Source: CAD feature listing. Evaluate the final solid. Frame: model axes, mm. A direction names the side the tool comes from. Give positions to 0.01 mm unless a question says otherwise; leave off trailing zeros. Loops run counter-clockwise (first coordinate to the right, second up) from the corner with the lowest first, then second, coordinate; pieces in that order, holes last. Notation, with made-up numbers: (33.5, 35) - (74.5, 35) arc R22 cw to (74.5, 63) - close; hole circle Ø3 at (72, 8.25). An arc over 180 degrees is marked (long way). Write each question's results on one line, items separated by ' | '. Start each with the question number.
(1) Reachability of faces 4 (the cylindrical face through (27.614, -11.205, 221.613)), 5 (the cylindrical face through (-49.45, 23.86, -48.18)), 6 (the flat face through (-39, -49.763, 127)) from +Z, -Z, +X, -X, +Y, -Y: full face, straight path, thin tool, end or side. Return the list, or none.
(2) Cut plane B-B on x = 10.5. Give the number of separate pieces and of enclosed holes in the cut face, then the cut area to 3 significant figures.
(3) Contact query for flat-ended pins moving along their axis: pin 1 (10 mm diameter, centred on x = 24, z = 237.5, fed in from +Y); pin 2 (5 mm diameter, centred on y = -4, z = 168, fed in from +X); pin 3 (1 mm diameter, centred on x = 53.5, y = -15, fed in from +Z). Output: stop coordinate, or through.
(4) Material intervals for line 1 along X through (y, z) = (20, 156.5); line 2 along Z through (x, y) = (-36, -55); line 3 along X through (y, z) = (12, 121.5), sorted ascending. Write a range as [from, to].
(5) Pull-direction query (Y, two-part tool) for faces 1 (the flat face through (31.978, -11, 124)), 2 (the cylindrical face through (52.096, -13.097, -48.175)), 3 (the flat face through (-62.829, -68.294, -35.434)); classes: pulls with the +Y half, pulls with the -Y half, needs draft (parallel to the pull), parting line crosses it, or undercut.
(6) Cut plane A-A on z = 124.5. Return the cut outline in (x, y).
(7) Cut plane C-C on y = -2.5. Return the cut outline in (x, z), then the cut area to 3 significant figures.
from build123d import *

# Parameters (mm, degrees)
RESSALTO_EXTRUS_O1_DEPTH             = 250
ESCALA1_SCALE                        = 1.5
AL_VIOS_SUPERIOR_INFERIOR_DEPTH      = 0.1
AL_VIOS_SUPERIOR_INFERIOR_DEPTH_BACK = 265
AL_VIOS_SUPERIOR_INFERIOR_START      = -55
AL_VIO_CENTRAL_DEPTH                 = 342.991467302
ESBO_O7_R                            = 40
REBAIXO_ROLAMENTO_PAI_DEPTH          = 46
ESBO_O7_3_R                          = 25
REBAIXO_ROLAMENTO_FILHO_DEPTH        = 395.297005295
FURO_START                           = -329
FURO_EIXO_ARMA_FILHO_DEPTH           = 46
FUROS_POLIA_PAI_D                    = 8.5
FUROS_POLIA_PAI_DEPTH                = 27.5
FUROS_POLIA_PAI_CSINK_D              = 10.05
FUROS_POLIA_PAI_CSINK_ANGLE          = 90
FUROS_POLIA_PAI_TIP                  = 2.553657631
FUROS_POLIA_FILHO_D                  = 8.5
FUROS_POLIA_FILHO_DEPTH              = 27.5
FUROS_POLIA_FILHO_CSINK_D            = 10.05
FUROS_POLIA_FILHO_CSINK_ANGLE        = 90
FUROS_POLIA_FILHO_TIP                = 2.553657631


with BuildPart() as part:
    # Esboço1 → Ressalto-extrusão1 (new body)
    with BuildSketch(Plane.XY):
        with BuildLine():
            Line((64.316370752, 0), (63.337395385, -14))
            Line((63.337395385, -14), (54.810070893, -37.42863149))
            Line((54.810070893, -37.42863149), (-37.189929107, -52))
            Line((-37.189929107, -52), (-49.547157766, -47.50233659))
            Line((-49.547157766, -47.50233659), (-58, -37.42863149))
            Line((-58, -37.42863149), (-58, 9.144452309))
            Line((-58, 9.144452309), (-49.934391816, 20.66333456))
            Line((-49.934391816, 20.66333456), (-37.189929107, 26.60617512))
            Line((-37.189929107, 26.60617512), (29.770815295, 20.747869084))
            Line((29.770815295, 20.747869084), (35.181577398, 9.144452309))
            ThreePointArc((35.181577398, 9.144452309), (42.631493482, 1.085178494), (53.376629903, -1.149813096))
            Line((53.376629903, -1.149813096), (64.316370752, 0))
        make_face()
    extrude(amount=RESSALTO_EXTRUS_O1_DEPTH)


with BuildPart() as part_1:
    # Escala1: scaled about (-4.187287107, -12.759804583, 125)
    add(part.part.scale(ESCALA1_SCALE).moved(Location((2.093643554, 6.379902291, -62.5))))

    # Esboço4 → Alívios superior / inferior (cut, two sides: drawn at the far end of the back side and taken through both)
    with BuildSketch(Plane(origin=(0, 0, -62.5), x_dir=(-1, 0, 0), z_dir=(0, 0, -1)).offset(AL_VIOS_SUPERIOR_INFERIOR_START - AL_VIOS_SUPERIOR_INFERIOR_DEPTH_BACK)):
        Polygon((-46.749866496, 37.501705917), (-51.978360206, 26.289164972), (80.570262297, 26.289164972), (72.807944171, 37.374904131), (53.691250107, 46.289164972), align=None)
        Polygon((72.227093095, -64.873602594), (84.906356446, -49.763044944), (-84.308749893, -49.763044944), (53.691250107, -71.620097709), align=None)
    extrude(amount=AL_VIOS_SUPERIOR_INFERIOR_DEPTH + AL_VIOS_SUPERIOR_INFERIOR_DEPTH_BACK, mode=Mode.SUBTRACT)

    # Esboço15 → Alívio Central (cut, through all)
    with BuildSketch(Plane(origin=(0, 26.289164972, 0), x_dir=(1, 0, 0), z_dir=(0, 1, 0))):
        with BuildLine():
            Line((-10.570262297, -17.4), (6.978360206, -17.4))
            ThreePointArc((6.978360206, -17.4), (24.656029736, -24.72233047), (31.978360206, -42.4))
            Line((31.978360206, -42.4), (31.978360206, -207.5))
            ThreePointArc((31.978360206, -207.5), (24.656029736, -225.17766953), (6.978360206, -232.5))
            Line((6.978360206, -232.5), (-10.570262297, -232.5))
            ThreePointArc((-10.570262297, -232.5), (-28.247931827, -225.17766953), (-35.570262297, -207.5))
            Line((-35.570262297, -207.5), (-35.570262297, -42.4))
            ThreePointArc((-35.570262297, -42.4), (-28.247931827, -24.72233047), (-10.570262297, -17.4))
        make_face()
    extrude(amount=-AL_VIO_CENTRAL_DEPTH, mode=Mode.SUBTRACT)

    # Esboço7 → Rebaixo rolamento (Pai) (cut)
    with BuildSketch(Plane.XY.offset(312.5)):
        with Locations((-1.158298377, -13.283920248)):
            Circle(ESBO_O7_R)
    extrude(amount=-REBAIXO_ROLAMENTO_PAI_DEPTH, mode=Mode.SUBTRACT)

    # Esboço7<3> → Rebaixo rolamento (Filho) (cut, through all)
    with BuildSketch(Plane.XY.offset(312.5)):
        with Locations((-1.158298377, -13.283920248)):
            Circle(ESBO_O7_3_R)
    extrude(amount=-REBAIXO_ROLAMENTO_FILHO_DEPTH, mode=Mode.SUBTRACT)

    # Esboço7 → Furo eixo arma (Filho) (cut)
    with BuildSketch(Plane.XY.offset(312.5).offset(FURO_START)):
        with Locations((-1.158298377, -13.283920248)):
            Circle(ESBO_O7_R)
    extrude(amount=-FURO_EIXO_ARMA_FILHO_DEPTH, mode=Mode.SUBTRACT)

    # Furos Polia (Pai)
    with Locations(Plane.XY.offset(312.5)):
        with Locations((56.341701623, -13.283920248), (-45.205853857, 23.676367309), (-58.623505242, -11.283920248), (-48.259540924, -46.264565338), (51.370565437, -36.671277225)):
            CounterSinkHole(FUROS_POLIA_PAI_D / 2, FUROS_POLIA_PAI_CSINK_D / 2, depth=FUROS_POLIA_PAI_DEPTH, counter_sink_angle=FUROS_POLIA_PAI_CSINK_ANGLE)
            with Locations((0, 0, -(FUROS_POLIA_PAI_DEPTH + FUROS_POLIA_PAI_TIP / 2))):  # 118° drill point
                Cone(0, FUROS_POLIA_PAI_D / 2, FUROS_POLIA_PAI_TIP, mode=Mode.SUBTRACT)

    # Furos Polia (Filho)
    with Locations(Plane(origin=(0, 0, -62.5), x_dir=(-1, 0, 0), z_dir=(0, 0, -1))):
        with Locations((45.205853857, 23.676367309), (58.623505242, -11.283920248), (48.259540924, -46.264565338), (-51.370565437, -36.671277225), (-56.341701623, -13.283920248)):
            CounterSinkHole(FUROS_POLIA_FILHO_D / 2, FUROS_POLIA_FILHO_CSINK_D / 2, depth=FUROS_POLIA_FILHO_DEPTH, counter_sink_angle=FUROS_POLIA_FILHO_CSINK_ANGLE)
            with Locations((0, 0, -(FUROS_POLIA_FILHO_DEPTH + FUROS_POLIA_FILHO_TIP / 2))):  # 118° drill point
                Cone(0, FUROS_POLIA_FILHO_D / 2, FUROS_POLIA_FILHO_TIP, mode=Mode.SUBTRACT)


solid = part_1.part
Ans:
1) face 4: +Y, -Y | face 5: -Z | face 6: +X, -X, -Y
2) separate pieces: 4 | enclosed holes: 0 | area: 5,000 mm^2
3) pin 1: y = 26.29 | pin 2: x = 98.02 | pin 3: z = 284.74
4) line 1: [-84.91, -35.57], [31.98, 54.91] | line 2: [-62.5, -7.6], [257.5, 312.5] | line 3: [-84.91, -35.57], [31.98, 60.67]
5) face 1: needs draft | face 2: undercut | face 3: pulls with the -Y half
6) outline: (-84.91, -49.76) - (-35.57, -49.76) - (-35.57, 26.29) - (-80.57, 26.29) - (-84.91, 20.1) - close; (31.98, -49.76) - (84.31, -49.76) - (97.1, -14.62) - (98.57, 6.38) - (82.16, 4.66) arc R27 cw to (54.87, 20.1) - (51.98, 26.29) - (31.98, 26.29) - close
7) outline: (-84.91, -62.5) - (-39.68, -62.5) - (-39.68, -16.5) - (-23.71, -16.5) - (-23.71, 21.13) arc R25 cw to (-35.57, 42.4) - (-35.57, 207.5) arc R25 cw to (-23.71, 228.77) - (-23.71, 266.5) - (-39.68, 266.5) - (-39.68, 312.5) - (-84.91, 312.5) - close; (21.4, -16.5) - (37.36, -16.5) - (37.36, -62.5) - (97.95, -62.5) - (97.95, 312.5) - (37.36, 312.5) - (37.36, 266.5) - (21.4, 266.5) - (21.4, 227.92) arc R25 cw to (31.98, 207.5) - (31.98, 42.4) arc R25 cw to (21.4, 21.98) - close | area: 44,400 mm^2
